from build123d import *

# Parameters (mm, degrees)
F0_R        = 2.5
F1_DEPTH    = 10
F2_R        = 2.15
F3_DEPTH    = 25
F5_T1_DEPTH = 10


# Not quite as in the source:
# - a fillet or chamfer that OpenCascade refuses, or shapes differently, is made with other operations: its cross-section is extruded or revolved along the edge and cut away or added


with BuildPart() as f1:
    # F0 (on Top) → F1 (new body)
    with BuildSketch(Plane.XY):
        with BuildLine():
            ThreePointArc((1.6, 5.2621288468), (5.4402071954, -0.8087927246), (0, -5.5))
            Line((0, -5.5), (0, -8))
            ThreePointArc((0, -8), (0.5345278854, -7.982122521), (1.0666667681, -7.9285699849))
            ThreePointArc((1.0666667681, -7.9285699849), (7.426445373, -2.9745435149), (6.2449979984, 5))
            ThreePointArc((6.2449979984, 5), (5.477264575, 5.8309152605), (4.6, 6.5452272688))
            ThreePointArc((4.6, 6.5452272688), (3.166710076, 7.3465602355), (1.6, 7.8383671769))
            Line((1.6, 7.8383671769), (1.6, 5.2621288468))
        make_face()
        with BuildLine():
            ThreePointArc((6.2449979984, 5), (7.426445373, -2.9745435149), (1.0666667681, -7.9285699849))
            Line((1.0666667681, -7.9285699849), (15.8, -5.9464274989))
            ThreePointArc((15.8, -5.9464274989), (9.0476534506, -0.7546989834), (14.2906457894, 5.9579204932))
            Line((14.2906457894, 5.9579204932), (6.2449979984, 5))
        make_face()
        with BuildLine():
            Line((1.6, 15), (1.6, 7.8383671769))
            ThreePointArc((1.6, 7.8383671769), (3.166710076, 7.3465602355), (4.6, 6.5452272688))
            Line((4.6, 6.5452272688), (4.6, 15))
            Line((4.6, 15), (1.6, 15))
        make_face()
        with BuildLine():
            ThreePointArc((14.2906457894, 5.9579204932), (9.0476534506, -0.7546989834), (15.8, -5.9464274989))
            ThreePointArc((15.8, -5.9464274989), (19.5166359163, -3.9496835316), (21, 0))
            ThreePointArc((21, 0), (18.9839600109, 4.4864309458), (14.2906457894, 5.9579204932))
        make_face()
        with Locations((15, 0)):
            Circle(F0_R, mode=Mode.SUBTRACT)
    extrude(amount=F1_DEPTH)

    # F2 (on face) → F3 (cut)
    with BuildSketch(Plane.YZ.offset(4.6)):
        with Locations((10.5, 5)):
            Circle(F2_R)
    extrude(amount=-F3_DEPTH, mode=Mode.SUBTRACT)

    # F4: F1 across plane


with BuildPart() as f1_1:
    add(f1.part)
    add(f1.part.mirror(Plane.YZ))

    # F5: fillet of radius 3.2 on 4 edges, made by hand

    # F5_s2 → F5_t1 (join)
    with BuildSketch(Plane.XY):
        with BuildLine():
            ThreePointArc((-5.5714285714, 5.7410089421), (-4.8528464095, 6.790702563), (-4.6, 8.037412519))
            Line((-4.6, 8.037412519), (-4.6, 6.5452272688))
            ThreePointArc((-4.6, 6.5452272688), (-5.1015861823, 6.1622900309), (-5.5714285714, 5.7410089421))
        make_face()
        with BuildLine():
            ThreePointArc((-7.8251476511, 5.1881337307), (-6.4876416555, 5.3128293037), (-5.3191610039, 5.9754938051))
            ThreePointArc((-5.3191610039, 5.9754938051), (-5.8026149621, 5.5072370206), (-6.2449979984, 5))
            Line((-6.2449979984, 5), (-7.8251476511, 5.1881337307))
        make_face()
        with BuildLine():
            ThreePointArc((7.8251476511, 5.1881337307), (6.4876416555, 5.3128293037), (5.3191610039, 5.9754938051))
            ThreePointArc((5.3191610039, 5.9754938051), (5.8026149621, 5.5072370206), (6.2449979984, 5))
            Line((6.2449979984, 5), (7.8251476511, 5.1881337307))
        make_face()
        with BuildLine():
            ThreePointArc((5.5714285714, 5.7410089421), (4.8528464095, 6.790702563), (4.6, 8.037412519))
            Line((4.6, 8.037412519), (4.6, 6.5452272688))
            ThreePointArc((4.6, 6.5452272688), (5.1015861823, 6.1622900309), (5.5714285714, 5.7410089421))
        make_face()
    extrude(amount=F5_T1_DEPTH)


solid = f1_1.part
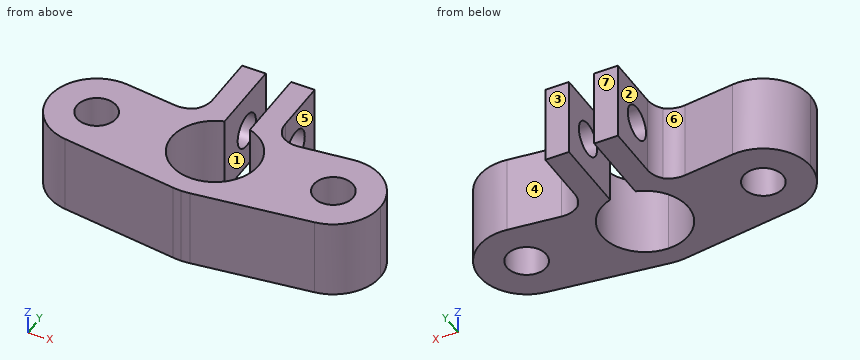
Work out the finished part from the listing and answer in its coordinate system (mm). Face numbers are marked on the shaded views. A direction names the side the tool comes from. Coordinates: 2 decimals unless noted, no trailing zeros. Write each loop counter-clockwise with the first axis right and the second up, starting at its lowest first coordinate (ties: lowest second). Pieces come first, ordered by that corner, then holes.
1. The part is cut by section C-C, the plane x = 16.5. Write down the section's boundary in (y, z).
Results list:
outline: (-5.81, 0) - (-2, 0) - (-2, 10) - (-5.81, 10) - close; (2, 0) - (5.81, 0) - (5.81, 10) - (2, 10) - close
2. The part is cut by section D-D, the plane z = 1.5. Write down the section's boundary in (x, y).
Results list:
outline: (-15.8, -5.95) - (-1.07, -7.93) arc R8 ccw to (1.07, -7.93) - (15.8, -5.95) arc R6 ccw to (14.29, 5.96) - (7.83, 5.19) arc R3.2 cw to (5.45, 5.86) arc R3.2 cw to (4.6, 8.04) - (4.6, 15) - (1.6, 15) - (1.6, 5.26) arc R5.5 cw (long way) to (-1.6, 5.26) - (-1.6, 15) - (-4.6, 15) - (-4.6, 8.04) arc R3.2 cw to (-5.45, 5.86) arc R3.2 cw to (-7.83, 5.19) - (-14.29, 5.96) arc R6 ccw to start; hole circle Ø5 at (-15, 0); hole circle Ø5 at (15, 0)
3. The part is cut by section A-A, the plane z = 3.75. Write down the section's boundary in (x, y).
Results list:
outline: (-15.8, -5.95) - (-1.07, -7.93) arc R8 ccw to (1.07, -7.93) - (15.8, -5.95) arc R6 ccw to (14.29, 5.96) - (7.83, 5.19) arc R3.2 cw to (5.45, 5.86) arc R3.2 cw to (4.6, 8.04) - (4.6, 8.75) - (1.6, 8.75) - (1.6, 5.26) arc R5.5 cw (long way) to (-1.6, 5.26) - (-1.6, 8.75) - (-4.6, 8.75) - (-4.6, 8.04) arc R3.2 cw to (-5.45, 5.86) arc R3.2 cw to (-7.83, 5.19) - (-14.29, 5.96) arc R6 ccw to start; (-4.6, 12.25) - (-1.6, 12.25) - (-1.6, 15) - (-4.6, 15) - close; (1.6, 12.25) - (4.6, 12.25) - (4.6, 15) - (1.6, 15) - close; hole circle Ø5 at (-15, 0); hole circle Ø5 at (15, 0)
4. For the marked faces 1, 2 and 3, determine the directions among +Z, -Z, +X, -X, +Y, -Y from which every point of the face is accessible in a straight line to the end or side of a thin tool.
Results list:
face 1: +Z, -Z, +Y
face 2: +Z, -Z, -X, +Y
face 3: +Z, -Z, +X, -X, +Y
5. For a pull along X with two mould halves and no side action, classify the marked faces 4, 5, 6 and 7 as +X half, -X half, draft (parallel to the pull), parting line (faces both ways), or undercut.
Results list:
face 4: undercut
face 5: +X half
face 6: undercut
face 7: draft
6. Consider line 1 along Z through (x, y) = (3.3, 10.5); line 2 along X through (y, z) = (1.75, 8); line 3 along X through (y, z) = (-4.5, 2). Determine where each line is inside the solid, lowest interval first.
Results list:
line 1: z = 0 to 2.85, 7.15 to 10
line 2: x = -20.74 to -16.79, -13.21 to -5.21, 5.21 to 13.21, 16.79 to 20.74
line 3: x = -18.97 to -3.16, 3.16 to 18.97
7. The part is cut by section B-B, the plane y = 3.75. Write down the section's boundary in (x, z), and give its area (3 significant figures).
Results list:
outline: (-19.68, 0) - (-4.02, 0) - (-4.02, 10) - (-19.68, 10) - close; (4.02, 0) - (19.68, 0) - (19.68, 10) - (4.02, 10) - close
area: 313 mm2
8. Flat-ended cylindrical pins translate along their axes: pin 1 (1 mm diameter, centred on x = -8.5, y = 5, fed in from -Z); pin 2 (3 mm diameter, centred on y = 5.5, z = 9, fed in from -X); pin 3 (3 mm diameter, centred on y = 11.5, z = 8.5, fed in from -X); pin 4 (2 mm diameter, centred on y = 4.5, z = 9, fed in from -X). Find the tip coordinate at first contact, or state that the pin passes through.
Results list:
pin 1: stops at z = 0
pin 2: stops at x = -19.47
pin 3: stops at x = -4.6
pin 4: stops at x = -19.87
